```python
from build123d import *

# Parameters (mm, degrees)
F1_DEPTH = 127
F2_R     = 3.2258
F3_DEPTH = 19.431


with BuildPart() as f1:
    # F0 (on Top) → F1 (new body)
    with BuildSketch(Plane.XY):
        Polygon((0, 19.431), (0, 0), (51.6382, 0), (110.60591, 0), (110.60591, 19.431), align=None)
        Polygon((110.60591, 0), (51.6382, 0), (51.6382, -22.86), (55.4482, -22.86), (55.4482, -2.794), (110.60591, -2.794), align=None)
    extrude(amount=F1_DEPTH)

    # F2 (on face) → F3 (cut, through all)
    with BuildSketch(Plane(origin=(0, 19.431, 0), x_dir=(-1, 0, 0), z_dir=(0, 1, 0))):
        with Locations((-34.036, 63.5)):
            Circle(F2_R)
    extrude(amount=-F3_DEPTH, mode=Mode.SUBTRACT)


solid = f1.part
```
Source: CAD feature listing. Evaluate the final solid. Frame: model axes, mm. A direction names the side the tool comes from. Coordinates: 2 decimals unless noted, no trailing zeros. Order: outer loops, then holes, each group sorted by start corner. A loop starts at its lowest first (then second) coordinate and runs counter-clockwise, first axis right, second up. Notation, with made-up numbers: M 77,19.25 L 83,19.25 A37 cw 83,58.25 Z; hole C -37.5,56 d11. An arc over 180 degrees is marked long. Write each question's results on one line, items separated by ' | '. Start each with the question number.
1) Draft query along Z for faces 1 (the face through (110.606, 8, 63)), 2 (the face through (34.74, 9.85, 60.35)), 3 (the face through (55, 8, 127)). Return one class per face: released by +Z, released by -Z, zero draft, split by the parting line, or undercut.
2) Section query A-A (z = 63.5). Return the cut outline in (x, y), plus the area to 3 significant figures.
3) Access query for faces 4 (the face through (54, -22.86, 63)), 5 (the face through (55.448, -13, 63)), 6 (the face through (25, 0, 63)). Directions: +Z, -Z, +X, -X, +Y, -Y. A direction counts if a zero-diameter tool reaches every point of the face in a straight line with its end or side. Return the directions, or none.
4) Line query: line 1 (Y direction, x = 45, z = 59); line 2 (Y direction, x = 60, z = 52); line 3 (X direction, y = -1.5, z = 14.5). Output: solid intervals per line, ascending. Write a range as from..to.
5) Section query C-C (x = 39.5). Return the cut outline in (y, z).
6) Section query B-B (z = 100). Return the cut outline in (x, y), plus the area to 3 significant figures.
7) Section query D-D (y = -20). Return the cut outline in (x, z), plus the area to 3 significant figures.
8) Contact query for flat-ended pins moving along their axis: pin 1 Ø5 at (y, z) = (-17.5, 27) entering from +X; pin 2 Ø15.5 at (x, z) = (16, 94.5) entering from -Y; pin 3 Ø7 at (y, z) = (-14.5, 73) entering from -X. Output: stop coordinate, or through.
Answers:
1) face 1: zero draft | face 2: undercut | face 3: released by +Z
2) outline: M 0,0 L 30.81,0 L 30.81,19.43 L 0,19.43 Z; M 37.26,0 L 51.64,0 L 51.64,-22.86 L 55.45,-22.86 L 55.45,-2.79 L 110.61,-2.79 L 110.61,19.43 L 37.26,19.43 Z | area: 2,270 mm^2
3) face 4: +Z, -Z, +X, -X, -Y | face 5: +Z, -Z, +X, -Y | face 6: +Z, -Z, -X, -Y
4) line 1: y = 0..19.43 | line 2: y = -2.79..19.43 | line 3: x = 51.64..110.61
5) outline: M 0,0 L 19.43,0 L 19.43,127 L 0,127 Z
6) outline: M 0,0 L 51.64,0 L 51.64,-22.86 L 55.45,-22.86 L 55.45,-2.79 L 110.61,-2.79 L 110.61,19.43 L 0,19.43 Z | area: 2,390 mm^2
7) outline: M 51.64,0 L 55.45,0 L 55.45,127 L 51.64,127 Z | area: 484 mm^2
8) pin 1: stops at x = 55.45 | pin 2: stops at y = 0 | pin 3: stops at x = 51.64
